Autodesk Inventor part; units mm, degrees
ref_plane "YZ Plane" through (0, 0, 0) normal (1, 0, 0) x (0, 1, 0)
ref_plane "XZ Plane" through (0, 0, 0) normal (0, 1, 0) x (-1, 0, 0)
ref_plane "XY Plane" through (0, 0, 0) normal (0, 0, 1) x (1, 0, 0)
sketch "Sketch1" plane through (0, 0, 0) normal (0, 1, 0) x (-1, 0, 0)
  line L0 (0, 0) -> (-22.8, 0)
  line L1 (-22.8, 0) -> (-22.8, -18)
  line L2 (-22.8, -18) -> (0, -18)
  line L3 (0, -18) -> (0, 0)
  dimension "d0" = 22.8
  dimension "d1" = 18
extrude "Extrusion1" add sketch "Sketch1" along normal blind 0.9
sketch "Sketch2" plane through (0, 0.9, 0) normal (0, 1, 0) x (1, 0, 0)
  line L0 (14.1431, 3.3431) -> (8.4863, 9)
  line L1 (8.4863, 9) -> (14.1431, 14.6569)
  line L2 (14.1431, 14.6569) -> (19.8, 9)
  line L3 (19.8, 9) -> (14.1431, 3.3431)
  line L4 (22.8, 0) -> (22.8, 18)
  point P0 (0, 0)
  point P1 (22.8, 9)
  dimension "d4" = 135
  dimension "d5" = 8
  dimension "d6" = 3
extrude "Extrusion2" add sketch "Sketch2" along normal blind 1
sketch "Sketch3" plane through (0, 0.9, 0) normal (0, 1, 0) x (1, 0, 0)
  line L0 (6, 4.5) -> (-1, 4.5)
  line L1 (-1, 4.5) -> (-1, 13.5)
  line L2 (-1, 13.5) -> (6, 13.5)
  line L3 (6, 13.5) -> (6, 4.5)
  line L4 (0, 18) -> (0, 0)
  point P0 (-1, 9)
  point P1 (0, 9)
  dimension "d9" = 7
  dimension "d10" = 1
  dimension "d11" = 9
extrude "Extrusion3" add sketch "Sketch3" along normal blind 3.2
fillet "Fillet1" radius 1.6 4 edges at (2.5, 4.1, -4.5) (2.5, 4.1, -13.5) (-0.5, 0.9, -4.5) (-0.5, 0.9, -13.5)
properties part number "rp2040"
The model under review builds one solid part; all positions refer to its coordinate system, in mm. A direction names the side the tool comes from. Round coordinates to 2 decimals unless told otherwise and drop trailing zeros. Loops run counter-clockwise (first coordinate to the right, second up) from the corner with the lowest first, then second, coordinate; pieces in that order, holes last. Notation, with made-up numbers: M 81,24 L 87,24 A9 cw 87,28 Z; hole C 78.25,82 d10. An arc over 180 degrees is marked long. Answer as CSV lines item,"result".
1. For faces 4 (the face through (2, 2, -13.5)), 5 (the face through (-0.5, 0.9, -9)), 6 (the face through (-0.493, 1.381, -4.956)), 7 (the face through (3, 2, -4.5)), list the 3-axis set-ups (+Z, -Z, +X, -X, +Y, -Y) from which the entire face can be reached by the end or side of a thin tool; tool diameter is ignored.
Outcome:
face 4,"-Z, -X, +Y"
face 5,"+Z, -Z, -X, -Y"
face 6,"+Z, -X, -Y"
face 7,"+Z, -X, +Y"
2. We need section B-B (z = -11). Give the boundary of the cut face in (x, y).
Outcome:
outline,"M -1,0.9 L 0,0.9 L 0,0 L 22.8,0 L 22.8,0.9 L 17.8,0.9 L 17.8,1.9 L 10.49,1.9 L 10.49,0.9 L 6,0.9 L 6,4.1 L -1,4.1 Z"
3. Insertion check: pin 1 Ø1 at (y, z) = (2, -7.5) entering from +X; pin 2 Ø2 at (x, y) = (17, 3.5) entering from +Z; pin 3 Ø1.3 at (x, y) = (3.5, 2) entering from +Z; pin 4 Ø1 at (y, z) = (1.5, -7) entering from +X. Each pin has a flat end and moves straight along its axis. Give the tip position at first contact, or say it passes through.
Outcome:
pin 1,"stops at x = 18.79"
pin 2,"passes through"
pin 3,"stops at z = -4.5"
pin 4,"stops at x = 18.3"
4. We need section A-A (x = 4). Give the boundary of the cut face in (y, z), plus the area to 3 significant figures.
Outcome:
outline,"M 0,-18 L 0.9,-18 L 0.9,-13.5 L 2.5,-13.5 A1.6 ccw 4.1,-11.9 L 4.1,-6.1 A1.6 ccw 2.5,-4.5 L 0.9,-4.5 L 0.9,0 L 0,0 Z"
area,"43.9 mm2"
5. We need section D-D (x = 17.75). Give the boundary of the cut face in (y, z).
Outcome:
outline,"M 0,-18 L 0.9,-18 L 0.9,-11.05 L 1.9,-11.05 L 1.9,-6.95 L 0.9,-6.95 L 0.9,0 L 0,0 Z"
6. We need section C-C (y = 0.3). Give the boundary of the cut face in (x, z).
Outcome:
outline,"M 0,-18 L 22.8,-18 L 22.8,0 L 0,0 Z"
7. Draft analysis for pull direction X (two halves, no side actions). For faces 1 (the face through (16.9, 1.4, -11.9)), 2 (the face through (6, 2, -9)), 3 (the face through (12, 0, -9)), state which applies: pulls with the +X half, pulls with the -X half, needs draft (parallel to the pull), parting line crosses it, or undercut.
Outcome:
face 1,"pulls with the +X half"
face 2,"undercut"
face 3,"needs draft"
8. To check wall thickness, follow L1, parallel to Y at x = 20, z = -13.75; L2, parallel to X at y = 0.6, z = -3.25; L3, parallel to X at y = 3.55, z = -8.5. State the ranges of each line that lie inside material, in increasing order. Write a range as [from, to].
Outcome:
L1,"y = [0, 0.9]"
L2,"x = [0, 22.8]"
L3,"x = [-1, 6]"
